Geometry check sheet. Reference: the model listing, model coordinates, mm. Give positions to 0.01 mm unless a question says otherwise; leave off trailing zeros. Loops run counter-clockwise (first coordinate to the right, second up) from the corner with the lowest first, then second, coordinate; pieces in that order, holes last. Notation, with made-up numbers: (-9.5, 30.5) -> (48.5, 30.5) arc R8 cw to (48.5, 42.5) -> close; hole circle Ø11 at (46, 10.5). An arc over 180 degrees is marked (long way). Write item = value, one per line. Start each with the question number.
```python
from build123d import *

# Parameters (mm, degrees)
BOSS_EXTRUDE2_DEPTH = 3
CUT_EXTRUDE4_DEPTH  = 10
SKETCH8_R           = 1
CUT_EXTRUDE5_DEPTH  = 10
SKETCH6_R           = 1.5
CUT_EXTRUDE6_DEPTH  = 10
CUT_EXTRUDE2_DEPTH  = 3
SKETCH5_R           = 1
CUT_EXTRUDE3_DEPTH  = 3


with BuildPart() as part:
    # Sketch2 → Boss-Extrude2 (new body)
    with BuildSketch(Plane(origin=(0, 0, 0), x_dir=(1, 0, 0), z_dir=(0, 1, 0))):
        with BuildLine():
            Line((-100, 58.061579531), (0, 48))
            ThreePointArc((0, 48), (24, 24), (0, 0))
            Line((0, 0), (-100, -11.145771569))
            ThreePointArc((-100, -11.145771569), (-134.60367555, 23.457903981), (-100, 58.061579531))
        make_face()
    extrude(amount=BOSS_EXTRUDE2_DEPTH)

    # Sketch7 → Cut-Extrude4 (cut)
    with BuildSketch(Plane(origin=(0, 3, 0), x_dir=(1, 0, 0), z_dir=(0, 1, 0))):
        with BuildLine():
            Line((5.344155686, 26.5), (5.904155686, 26.5))
            ThreePointArc((5.904155686, 26.5), (8.404155686, 24), (5.904155686, 21.5))
            Line((5.904155686, 21.5), (5.344155686, 21.5))
            ThreePointArc((5.344155686, 21.5), (-5.9, 24), (5.344155686, 26.5))
        make_face()
    extrude(amount=-CUT_EXTRUDE4_DEPTH, mode=Mode.SUBTRACT)

    # Sketch8 → Cut-Extrude5 (cut)
    with BuildSketch(Plane(origin=(0, 3, 0), x_dir=(1, 0, 0), z_dir=(0, 1, 0))):
        with Locations(Location((-9.2, 24, 0), (0, 0, 270))):
            Circle(SKETCH8_R)
    extrude(amount=-CUT_EXTRUDE5_DEPTH, mode=Mode.SUBTRACT)

    # Sketch6 → Cut-Extrude6 (cut)
    with BuildSketch(Plane(origin=(0, 3, 0), x_dir=(1, 0, 0), z_dir=(0, 1, 0))):
        with Locations(Location((-100, 23.457903981, 0), (0, 0, 270))):
            Circle(SKETCH6_R)
    extrude(amount=-CUT_EXTRUDE6_DEPTH, mode=Mode.SUBTRACT)

    # Sketch3 → Cut-Extrude2 (cut)
    with BuildSketch(Plane(origin=(0, 3, 0), x_dir=(1, 0, 0), z_dir=(0, 1, 0))):
        with BuildLine():
            Line((5.344155686, 26.5), (5.9, 26.5))
            ThreePointArc((5.9, 26.5), (8.4, 24), (5.9, 21.5))
            Line((5.9, 21.5), (5.344155686, 21.5))
            ThreePointArc((5.344155686, 21.5), (-5.9, 24), (5.344155686, 26.5))
        make_face()
    extrude(amount=-CUT_EXTRUDE2_DEPTH, mode=Mode.SUBTRACT)

    # Sketch5 → Cut-Extrude3 (cut)
    with BuildSketch(Plane(origin=(0, 3, 0), x_dir=(1, 0, 0), z_dir=(0, 1, 0))):
        with Locations((-9.3, 24)):
            Circle(SKETCH5_R)
    extrude(amount=-CUT_EXTRUDE3_DEPTH, mode=Mode.SUBTRACT)


solid = part.part
```
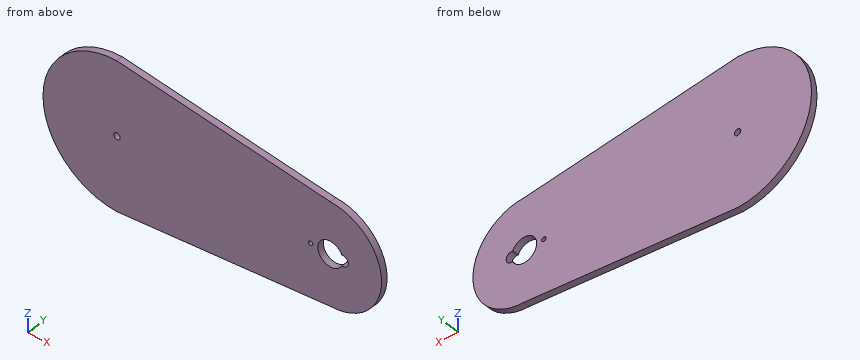
1) Section check A-A (y = 1.4). Enter the section's corners in (x, z).
2) Section check C-C (z = -9.5). Enter the section's corners in (x, y).
3) Thickness scan on line 1 (Z direction, x = -100, y = 1.55); line 2 (Z direction, x = 0, y = 0.9); line 3 (X direction, y = 1.95, z = -24). Record the ranges inside material, lowest first.
4) Section check B-B (x = -18). Enter the section's corners in (y, z).
5) Depth check by flat-ended pin: pin 1 Ø1.5 at (x, z) = (-87, -41) entering from -Y. Enter the tip coordinate at first touch or a pass-through.
Check result:
q1.outline = (-100, -58.06) -> (0, -48) arc R24 ccw to (0, 0) -> (-100, 11.15) arc R34.6 ccw to start; hole circle Ø3 at (-100, -23.46); hole (-9.25, -25) arc R1 ccw (long way) to (-9.25, -23) arc R1 ccw (long way) to start; hole (5.34, -26.5) -> (5.9, -26.5) arc R2.5 ccw to (5.9, -21.5) -> (5.34, -21.5) arc R5.9 ccw (long way) to start
q2.outline = (-131.66, 0) -> (19.12, 0) -> (19.12, 3) -> (-131.66, 3) -> close
q3.line_1 = -58.06 to -24.96, -21.96 to 11.15
q3.line_2 = -48 to -29.9, -18.1 to 0
q3.line_3 = -134.6 to -101.4, -98.6 to -10.3, -8.2 to -5.9, 8.4 to 24
q4.outline = (0, -49.81) -> (3, -49.81) -> (3, 2.01) -> (0, 2.01) -> close
q5.pin_1 = 0
